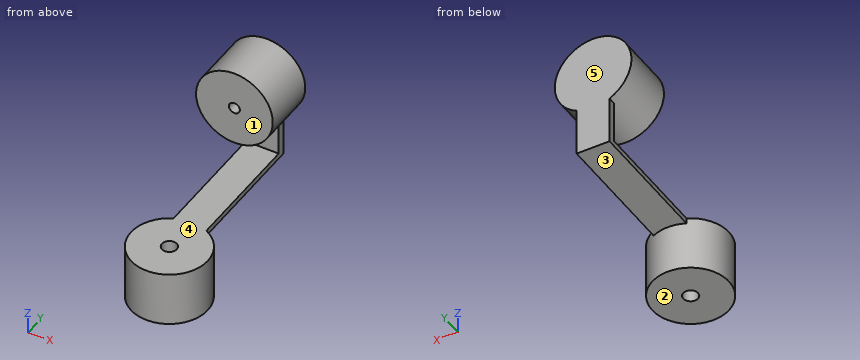
```python
from build123d import *

# Parameters (mm, degrees)
SKETCH1_R           = 35
BOSS_EXTRUDE1_DEPTH = 50
SKETCH2_W           = 30
SKETCH2_H           = 5
BOSS_EXTRUDE2_DEPTH = 150
SKETCH3_W           = 30
SKETCH3_H           = 7.079136618
BOSS_EXTRUDE3_DEPTH = 70
SKETCH5_R           = 35
BOSS_EXTRUDE4_DEPTH = 50
SKETCH6_R           = 6.791338944
CUT_EXTRUDE1_DEPTH  = 50
SKETCH7_R           = 5
CUT_EXTRUDE2_DEPTH  = 10


with BuildPart() as part:
    # Sketch1 → Boss-Extrude1 (new body)
    with BuildSketch(Plane.XY):
        Circle(SKETCH1_R)
    extrude(amount=BOSS_EXTRUDE1_DEPTH)

    # Sketch2 → Boss-Extrude2 (add)
    with BuildSketch(Plane(origin=(0, 0, 0), x_dir=(1, 0, 0), z_dir=(0, 1, 0))):
        with Locations((0, -47.5)):
            Rectangle(SKETCH2_W, SKETCH2_H)
    extrude(amount=BOSS_EXTRUDE2_DEPTH)

    # Sketch3 → Boss-Extrude3 (add)
    with BuildSketch(Plane.XY.offset(50)):
        with Locations((0, 146.460431691)):
            Rectangle(SKETCH3_W, SKETCH3_H)
    extrude(amount=BOSS_EXTRUDE3_DEPTH)

    # Sketch5 → Boss-Extrude4 (add)
    with BuildSketch(Plane(origin=(0, 150, 0), x_dir=(1, 0, 0), z_dir=(0, 1, 0))):
        with Locations(Location((0, -120, 0), (0, 0, 270))):
            Circle(SKETCH5_R)
    extrude(amount=-BOSS_EXTRUDE4_DEPTH)

    # Sketch6 → Cut-Extrude1 (cut)
    with BuildSketch(Plane(origin=(0, 0, 0), x_dir=(-1, 0, 0), z_dir=(0, 0, -1))):
        Circle(SKETCH6_R)
    extrude(amount=-CUT_EXTRUDE1_DEPTH, mode=Mode.SUBTRACT)

    # Sketch7 → Cut-Extrude2 (cut)
    with BuildSketch(Plane.XZ.offset(-100)):
        with Locations(Location((0, 120, 0), (0, 0, 270))):
            Circle(SKETCH7_R)
    extrude(amount=-CUT_EXTRUDE2_DEPTH, mode=Mode.SUBTRACT)


solid = part.part
```
Verification items for the finished model (mm, model axes). Face numbers are marked on the shaded views. A direction names the side the tool comes from. Give positions to 0.01 mm unless a question says otherwise; leave off trailing zeros. Loops run counter-clockwise (first coordinate to the right, second up) from the corner with the lowest first, then second, coordinate; pieces in that order, holes last.
1. Section check B-B, the plane x = 0. Enter the section's corners in (y, z).
2. Mould release check, pull along Z, two halves, no side actions. Record for the marked faces 3, 4 and 5: released by +Z, released by -Z, zero draft, split by the parting line, or undercut.
3. Go/stop test with flat-tipped pins: pin 1 Ø8 at (x, z) = (-21.5, 16) entering from +Y; pin 2 Ø15 at (x, z) = (-5, 63) entering from -Y; pin 3 Ø5 at (y, z) = (111.5, 137) entering from +X. Record where each tip stops, or that it passes through.
4. Set-up check for the marked faces 1 and 2: record each of +Z, -Z, +X, -X, +Y, -Y from which the full face is reachable in a straight line by a thin tool's end or side.
5. Section check A-A, the plane y = 0. Enter the section's corners in (x, z), then the cut area to 3 significant figures.
6. Section check C-C, the plane z = 120. Enter the section's corners in (x, y), then the cut area to 3 significant figures.
7. Section check D-D, the plane z = 23. Enter the section's corners in (x, y), then the cut area to 3 significant figures.
8. Thickness scan on line 1 (X direction, y = 103, z = 120); line 2 (Y direction, x = 0, z = 23.5); line 3 (Z direction, x = 14, y = 68). Record the ranges inside material, lowest first.
Geometry says:
1. outline: (-35, 0) - (-6.79, 0) - (-6.79, 50) - (-35, 50) - close; (6.79, 0) - (35, 0) - (35, 45) - (150, 45) - (150, 155) - (100, 155) - (100, 125) - (110, 125) - (110, 115) - (100, 115) - (100, 85) - (142.92, 85) - (142.92, 50) - (6.79, 50) - close
2. face 3: released by -Z
2. face 4: undercut
2. face 5: zero draft
3. pin 1: stops at y = 30.31
3. pin 2: stops at y = 142.92
3. pin 3: stops at x = 31.86
4. face 1: +Z, +X, -X, -Y
4. face 2: -Z, +X, -X, +Y, -Y
5. outline: (-35, 0) - (-6.79, 0) - (-6.79, 50) - (-35, 50) - close; (6.79, 0) - (35, 0) - (35, 50) - (6.79, 50) - close
5. area: 2,820 mm2
6. outline: (-35, 100) - (-5, 100) - (-5, 110) - (5, 110) - (5, 100) - (35, 100) - (35, 150) - (-35, 150) - close
6. area: 3,400 mm2
7. outline: circle Ø70 at (0, 0); hole circle Ø13.58 at (0, 0)
7. area: 3,700 mm2
8. line 1: x = -35 to -5, 5 to 35
8. line 2: y = -35 to -6.79, 6.79 to 35
8. line 3: z = 45 to 50
